from build123d import *

# Parameters (mm, degrees)
BOSS_EXTRUDE1_DEPTH = 2


with BuildPart() as part:
    # Sketch1 → Boss-Extrude1 (new body)
    with BuildSketch(Plane(origin=(0, 0, 0), x_dir=(1, 0, 0), z_dir=(0, 0, -1))):
        Polygon((1.99, 1.99), (0, 0), (0, -47), (173.13, -47), (173.13, 0), (171.14, 1.99), (171.14, 10), (173.13, 10), (173.13, 30), (0, 30), (0, 10), (1.99, 10), align=None)
        Polygon((7.96, 1.99), (5.97, 0), (3.98, 1.99), (3.98, 10), (7.96, 10), align=None, mode=Mode.SUBTRACT)
        Polygon((13.93, 1.99), (11.94, 0), (9.95, 1.99), (9.95, 10), (13.93, 10), align=None, mode=Mode.SUBTRACT)
        Polygon((19.9, 1.99), (17.91, 0), (15.92, 1.99), (15.92, 10), (19.9, 10), align=None, mode=Mode.SUBTRACT)
        Polygon((25.87, 1.99), (23.88, 0), (21.89, 1.99), (21.89, 10), (25.87, 10), align=None, mode=Mode.SUBTRACT)
        Polygon((31.84, 1.99), (29.85, 0), (27.86, 1.99), (27.86, 10), (31.84, 10), align=None, mode=Mode.SUBTRACT)
        Polygon((37.81, 1.99), (35.82, 0), (33.83, 1.99), (33.83, 10), (37.81, 10), align=None, mode=Mode.SUBTRACT)
        Polygon((43.78, 1.99), (41.79, 0), (39.8, 1.99), (39.8, 10), (43.78, 10), align=None, mode=Mode.SUBTRACT)
        Polygon((49.75, 1.99), (47.76, 0), (45.77, 1.99), (45.77, 10), (49.75, 10), align=None, mode=Mode.SUBTRACT)
        Polygon((55.72, 1.99), (53.73, 0), (51.74, 1.99), (51.74, 10), (55.72, 10), align=None, mode=Mode.SUBTRACT)
        Polygon((61.69, 1.99), (59.7, 0), (57.71, 1.99), (57.71, 10), (61.69, 10), align=None, mode=Mode.SUBTRACT)
        Polygon((67.66, 1.99), (65.67, 0), (63.68, 1.99), (63.68, 10), (67.66, 10), align=None, mode=Mode.SUBTRACT)
        Polygon((73.63, 1.99), (71.64, 0), (69.65, 1.99), (69.65, 10), (73.63, 10), align=None, mode=Mode.SUBTRACT)
        Polygon((79.6, 1.99), (77.61, 0), (75.62, 1.99), (75.62, 10), (79.6, 10), align=None, mode=Mode.SUBTRACT)
        Polygon((85.57, 1.99), (83.58, 0), (81.59, 1.99), (81.59, 10), (85.57, 10), align=None, mode=Mode.SUBTRACT)
        Polygon((91.54, 1.99), (89.55, 0), (87.56, 1.99), (87.56, 10), (91.54, 10), align=None, mode=Mode.SUBTRACT)
        Polygon((97.51, 1.99), (95.52, 0), (93.53, 1.99), (93.53, 10), (97.51, 10), align=None, mode=Mode.SUBTRACT)
        Polygon((103.48, 1.99), (101.49, 0), (99.5, 1.99), (99.5, 10), (103.48, 10), align=None, mode=Mode.SUBTRACT)
        Polygon((109.45, 1.99), (107.46, 0), (105.47, 1.99), (105.47, 10), (109.45, 10), align=None, mode=Mode.SUBTRACT)
        Polygon((115.42, 1.99), (113.43, 0), (111.44, 1.99), (111.44, 10), (115.42, 10), align=None, mode=Mode.SUBTRACT)
        Polygon((121.39, 1.99), (119.4, 0), (117.41, 1.99), (117.41, 10), (121.39, 10), align=None, mode=Mode.SUBTRACT)
        Polygon((127.36, 1.99), (125.37, 0), (123.38, 1.99), (123.38, 10), (127.36, 10), align=None, mode=Mode.SUBTRACT)
        Polygon((133.33, 1.99), (131.34, 0), (129.35, 1.99), (129.35, 10), (133.33, 10), align=None, mode=Mode.SUBTRACT)
        Polygon((139.3, 1.99), (137.31, 0), (135.32, 1.99), (135.32, 10), (139.3, 10), align=None, mode=Mode.SUBTRACT)
        Polygon((145.27, 1.99), (143.28, 0), (141.29, 1.99), (141.29, 10), (145.27, 10), align=None, mode=Mode.SUBTRACT)
        Polygon((151.24, 1.99), (149.25, 0), (147.26, 1.99), (147.26, 10), (151.24, 10), align=None, mode=Mode.SUBTRACT)
        Polygon((157.21, 1.99), (155.22, 0), (153.23, 1.99), (153.23, 10), (157.21, 10), align=None, mode=Mode.SUBTRACT)
        Polygon((163.18, 1.99), (161.19, 0), (159.2, 1.99), (159.2, 10), (163.18, 10), align=None, mode=Mode.SUBTRACT)
        Polygon((169.15, 1.99), (167.16, 0), (165.17, 1.99), (165.17, 10), (169.15, 10), align=None, mode=Mode.SUBTRACT)
    extrude(amount=BOSS_EXTRUDE1_DEPTH)


solid = part.part
Could you check a few things on this model? Use its own coordinates, in mm. Give positions to 0.01 mm unless a question says otherwise; leave off trailing zeros.
1. Suppose I cut it at A-A (y = -5). State how many separate pieces and enclosed holes the cut face has, plus the area to 3 significant figures.
Answers below:
separate pieces: 29
enclosed holes: 0
area: 115 mm2
2. I need wall thicknesses on L1, parallel to Y at x = 82, z = -1.85; L2, parallel to Y at x = 22, z = -1.4. Which ranges of each line are inside material? Lowest first, please.
Answers below:
L1: y = -30 to -10, -1.58 to 47
L2: y = -30 to -10, -1.88 to 47
3. For pin 1 (8 mm diameter, centred on x = 79, y = 23.5, fed in from +Z); pin 2 (1 mm diameter, centred on y = -7.5, z = -1, fed in from +X); pin 3 (0.6 mm diameter, centred on y = -7, z = -0.5, fed in from -X), each with a flat end and sliding along its axis, tell me the tip position at first contact or that it passes through.
Answers below:
pin 1: stops at z = 0
pin 2: stops at x = 171.14
pin 3: stops at x = 1.99
